Design review of the part built by this model. Coordinates are the model's own, in mm. A direction names the side the tool comes from. Coordinates: 2 decimals unless noted, no trailing zeros. Write each loop counter-clockwise with the first axis right and the second up, starting at its lowest first coordinate (ties: lowest second). Pieces come first, ordered by that corner, then holes. Notation, with made-up numbers: (10.5, 66) -> (30.5, 66) arc R14 ccw to (30.5, 80) -> close; hole circle Ø6 at (31, 52). An arc over 180 degrees is marked (long way). Return JSON: item names as keys, results as strings. Group by question number.
from build123d import *

# Parameters (mm, degrees)
SKETCH2_R                                     = 1.75
CUT_EXTRUDE1_DEPTH                            = 46.369317826
CIRPATTERN1_COUNT                             = 6
SKETCH5_OUTSIDE_W                             = 75.336
SKETCH5_OUTSIDE_H                             = 75.336
SKETCH5_OUTSIDE_R                             = 1.75
CUT_EXTRUDE2_DEPTH                            = 10
CIRPATTERN2_COUNT                             = 6
SKETCH6_R                                     = 12
CUT_EXTRUDE3_DEPTH                            = 4.5
CBORE_FOR_M3_HEX_HEAD_MACHINE_SCREW1_AT_COUNT = 2
CBORE_FOR_M3_HEX_HEAD_MACHINE_SCREW1_AT_PITCH = 23.25
CBORE_FOR_M3_HEX_HEAD_MACHINE_SCREW1_2_COUNT  = 2
CBORE_FOR_M3_HEX_HEAD_MACHINE_SCREW1_2_PITCH  = 40.270181276
CBORE_FOR_M3_HEX_HEAD_MACHINE_SCREW1_3_COUNT  = 2
CBORE_FOR_M3_HEX_HEAD_MACHINE_SCREW1_3_PITCH  = 46.5
CBORE_FOR_M3_HEX_HEAD_MACHINE_SCREW1_4_COUNT  = 2
CBORE_FOR_M3_HEX_HEAD_MACHINE_SCREW1_4_PITCH  = 40.270181276
CBORE_FOR_M3_HEX_HEAD_MACHINE_SCREW1_5_COUNT  = 2
CBORE_FOR_M3_HEX_HEAD_MACHINE_SCREW1_5_PITCH  = 23.25
SKETCH9_R                                     = 4.2
CUT_EXTRUDE4_DEPTH                            = 46.369317826
CIRPATTERN3_START                             = -26.5
CIRPATTERN3_DEPTH                             = 21.5


# Read off the part's stored shape, not the designer's step: CirPattern3
with BuildPart() as part:
    # Sketch1 → Revolve1 (revolve)
    with BuildSketch(Plane(origin=(0, 0, 0), x_dir=(0, 0, -1), z_dir=(1, 0, 0)), mode=Mode.PRIVATE) as revolve1_sk:
        Polygon((0, 0), (0, 28.25), (5, 28.25), (5, 24.5), (8.5, 24.5), (8.5, 22.5), (26.5, 22.5), (26.5, 0), align=None)
    revolve(revolve1_sk.sketch.rotate(Axis((0, 0, 0), (0, 0, -1)), 90), axis=Axis((0, 0, 0), (0, 0, -1)))

    # Sketch2 → Cut-Extrude1 (cut, symmetric)
    with BuildSketch(Plane(origin=(0, 0, -5), x_dir=(-1, 0, 0), z_dir=(0, 0, -1))):
        with Locations((0, 23.25)):
            Circle(SKETCH2_R)
    cut_extrude1 = extrude(amount=CUT_EXTRUDE1_DEPTH, both=True, mode=Mode.SUBTRACT)

    # CirPattern1: Cut-Extrude1 ×6 about axis
    cirpattern1_axis = Axis((0, 0, 0), (0, 0, 1))
    for i in range(1, CIRPATTERN1_COUNT):
        add(cut_extrude1.rotate(cirpattern1_axis, i * 360 / CIRPATTERN1_COUNT), mode=Mode.SUBTRACT)

    # Sketch5 outside → Cut-Extrude2 (cut)
    # profile 1 of 2: a face of its own
    with BuildSketch(Plane(origin=(0, 0, -26.5), x_dir=(-1, 0, 0), z_dir=(0, 0, -1))):
        Rectangle(SKETCH5_OUTSIDE_W, SKETCH5_OUTSIDE_H)
        with BuildLine():
            ThreePointArc((-1.554498096, 22.446236559), (-11.25, 19.485571585), (-18.661762031, 12.569353121))
            ThreePointArc((-18.661762031, 12.569353121), (-18.619546181, 10.75), (-20.216260128, 9.876883438))
            ThreePointArc((-20.216260128, 9.876883438), (-22.5, 0), (-20.216260128, -9.876883438))
            ThreePointArc((-20.216260128, -9.876883438), (-18.619546181, -10.75), (-18.661762031, -12.569353121))
            ThreePointArc((-18.661762031, -12.569353121), (-11.25, -19.485571585), (-1.554498096, -22.446236559))
            ThreePointArc((-1.554498096, -22.446236559), (0, -21.5), (1.554498096, -22.446236559))
            ThreePointArc((1.554498096, -22.446236559), (11.25, -19.485571585), (18.661762031, -12.569353121))
            ThreePointArc((18.661762031, -12.569353121), (18.619546181, -10.75), (20.216260128, -9.876883438))
            ThreePointArc((20.216260128, -9.876883438), (22.5, 0), (20.216260128, 9.876883438))
            ThreePointArc((20.216260128, 9.876883438), (18.619546181, 10.75), (18.661762031, 12.569353121))
            ThreePointArc((18.661762031, 12.569353121), (11.25, 19.485571585), (1.554498096, 22.446236559))
            ThreePointArc((1.554498096, 22.446236559), (0, 21.5), (-1.554498096, 22.446236559))
        make_face(mode=Mode.SUBTRACT)
    # profile 2 of 2: a face of its own
    with BuildSketch(Plane(origin=(0, 0, -26.5), x_dir=(-1, 0, 0), z_dir=(0, 0, -1))):
        with Locations((8.25, 14.289419162)):
            Circle(SKETCH5_OUTSIDE_R)
    cut_extrude2 = extrude(amount=-CUT_EXTRUDE2_DEPTH, mode=Mode.SUBTRACT)

    # CirPattern2: Cut-Extrude2 ×6 about axis
    cirpattern2_axis = Axis((0, 0, 0), (0, 0, 1))
    for i in range(1, CIRPATTERN2_COUNT):
        add(cut_extrude2.rotate(cirpattern2_axis, i * 360 / CIRPATTERN2_COUNT), mode=Mode.SUBTRACT)

    # Sketch6 → Cut-Extrude3 (cut)
    with BuildSketch(Plane.XY):
        Circle(SKETCH6_R)
    extrude(amount=-CUT_EXTRUDE3_DEPTH, mode=Mode.SUBTRACT)

    # Sketch8 → CBORE for M3 Hex Head Machine Screw1 (revolve, cut)
    with BuildSketch(Plane(origin=(20.135090638, 11.625, -5), x_dir=(0, 1, 0), z_dir=(1, 0, 0))):
        Polygon((0, 0), (0, 5), (1.7, 5), (1.7, 2.3), (4.2, 2.3), (4.2, 0), align=None)
    cbore_for_m3_hex_head_machine_screw1 = revolve(axis=Axis((20.135090638, 11.625, -11.35), (0, 0, 1)), mode=Mode.SUBTRACT)

    # CBORE for M3 Hex Head Machine Screw1 at: CBORE for M3 Hex Head Machine Screw1 ×2
    with Locations(*[Vector(-0.8660254037844417, 0.49999999999999484, 0) * (i * CBORE_FOR_M3_HEX_HEAD_MACHINE_SCREW1_AT_PITCH) for i in range(1, CBORE_FOR_M3_HEX_HEAD_MACHINE_SCREW1_AT_COUNT)]):
        add(cbore_for_m3_hex_head_machine_screw1, mode=Mode.SUBTRACT)

    # CBORE for M3 Hex Head Machine Screw1 2: CBORE for M3 Hex Head Machine Screw1 ×2
    with Locations(*[(-i * CBORE_FOR_M3_HEX_HEAD_MACHINE_SCREW1_2_PITCH, 0, 0) for i in range(1, CBORE_FOR_M3_HEX_HEAD_MACHINE_SCREW1_2_COUNT)]):
        add(cbore_for_m3_hex_head_machine_screw1, mode=Mode.SUBTRACT)

    # CBORE for M3 Hex Head Machine Screw1 3: CBORE for M3 Hex Head Machine Screw1 ×2
    with Locations(*[Vector(-0.8660254037844346, -0.5000000000000071, 0) * (i * CBORE_FOR_M3_HEX_HEAD_MACHINE_SCREW1_3_PITCH) for i in range(1, CBORE_FOR_M3_HEX_HEAD_MACHINE_SCREW1_3_COUNT)]):
        add(cbore_for_m3_hex_head_machine_screw1, mode=Mode.SUBTRACT)

    # CBORE for M3 Hex Head Machine Screw1 4: CBORE for M3 Hex Head Machine Screw1 ×2
    with Locations(*[Vector(-0.49999999999999495, -0.8660254037844416, 0) * (i * CBORE_FOR_M3_HEX_HEAD_MACHINE_SCREW1_4_PITCH) for i in range(1, CBORE_FOR_M3_HEX_HEAD_MACHINE_SCREW1_4_COUNT)]):
        add(cbore_for_m3_hex_head_machine_screw1, mode=Mode.SUBTRACT)

    # CBORE for M3 Hex Head Machine Screw1 5: CBORE for M3 Hex Head Machine Screw1 ×2
    with Locations(*[(0, -i * CBORE_FOR_M3_HEX_HEAD_MACHINE_SCREW1_5_PITCH, 0) for i in range(1, CBORE_FOR_M3_HEX_HEAD_MACHINE_SCREW1_5_COUNT)]):
        add(cbore_for_m3_hex_head_machine_screw1, mode=Mode.SUBTRACT)

    # Sketch9 → Cut-Extrude4 (cut, through all)
    with BuildSketch(Plane(origin=(0, 0, -5), x_dir=(-1, 0, 0), z_dir=(0, 0, -1))):
        with Locations((-20.135090638, 11.625)):
            Circle(SKETCH9_R)
    extrude(amount=CUT_EXTRUDE4_DEPTH, mode=Mode.SUBTRACT)

    # CirPattern3 outline → CirPattern3 (cut)
    with BuildSketch(Plane.XY.offset(CIRPATTERN3_START)):
        with BuildLine():
            ThreePointArc((-1.256823209, 24.467741935), (-2.811398825, 24.338160091), (-4.35457664, 24.109907969))
            ThreePointArc((-4.35457664, 24.109907969), (-0.179741778, 19.176685596), (3.901890218, 24.187295275))
            ThreePointArc((3.901890218, 24.187295275), (2.58316543, 24.363440979), (1.256823209, 24.467741935))
            ThreePointArc((1.256823209, 24.467741935), (0, 21.5), (-1.256823209, 24.467741935))
        make_face()
        with BuildLine():
            ThreePointArc((-18.968503996, 15.506316654), (-19.795032609, 14.436297449), (-20.561274485, 13.322311795))
            ThreePointArc((-20.561274485, 13.322311795), (-18.619546181, 10.75), (-21.818097694, 11.145430141))
            ThreePointArc((-21.818097694, 11.145430141), (-22.490778714, 9.716731593), (-23.070024017, 8.247665844))
            ThreePointArc((-23.070024017, 8.247665844), (-16.916681459, 9.558816026), (-18.968503996, 15.506316654))
        make_face()
        with BuildLine():
            ThreePointArc((-21.818097694, -11.145430141), (-18.619546181, -10.75), (-20.561274485, -13.322311795))
            ThreePointArc((-20.561274485, -13.322311795), (-19.723759912, -14.533523143), (-18.81499127, -15.692230674))
            ThreePointArc((-18.81499127, -15.692230674), (-16.935996673, -9.778002238), (-22.997366041, -8.448145074))
            ThreePointArc((-22.997366041, -8.448145074), (-22.448280204, -9.814515571), (-21.818097694, -11.145430141))
        make_face()
        with BuildLine():
            ThreePointArc((-1.256823209, -24.467741935), (0, -21.5), (1.256823209, -24.467741935))
            ThreePointArc((1.256823209, -24.467741935), (2.604684023, -24.361149832), (3.944612144, -24.180364659))
            ThreePointArc((3.944612144, -24.180364659), (-0.18016322, -19.429683905), (-4.392323866, -24.103059786))
            ThreePointArc((-4.392323866, -24.103059786), (-2.830452956, -24.335951513), (-1.256823209, -24.467741935))
        make_face()
        with BuildLine():
            ThreePointArc((20.561274485, -13.322311795), (18.619546181, -10.75), (21.818097694, -11.145430141))
            ThreePointArc((21.818097694, -11.145430141), (22.390941527, -9.944633606), (22.897757266, -8.714511586))
            ThreePointArc((22.897757266, -8.714511586), (16.517625997, -9.744003743), (18.702504464, -15.826127977))
            ThreePointArc((18.702504464, -15.826127977), (19.671765509, -14.603822849), (20.561274485, -13.322311795))
        make_face()
    extrude(amount=CIRPATTERN3_DEPTH, mode=Mode.SUBTRACT)


solid = part.part
Q1. For faces 4 (the flat face through (-23, 0, -8.5)), 5 (the flat face through (11, 20, -8.5)), 6 (the cylindrical face through (16.57, -9.66, -15.9)), 7 (the cylindrical face through (-11.267, -19.476, -17.626)), list the 3-axis set-ups (+Z, -Z, +X, -X, +Y, -Y) from which the entire face can be reached by the end or side of a thin tool; tool diameter is ignored.
Q2. We need section A-A on y = -23.25. Write out the cut boundary in (x, z).
Q3. We need section C-C on z = -23. State how many separate pieces and enclosed holes the cut face has, plus the area to 3 significant figures.
Q4. We need section D-D on x = -8.25. Write out the cut boundary in (y, z), plus the area to 3 significant figures.
Q5. For P1, Ø4, axis at y = -21.5, z = -22.5, coming from the -X side (3 decimals); P2, Ø12, axis at x = -0.5, y = -1, coming from the +Z side; P3, Ø4, axis at x = -1, y = -22, coming from the -Z side; P4, Ø2, axis at x = 20.14, y = 11.63, coming from the -Z side, all flat-tipped, find the tip position at first contact; note any pin that passes through.
Q6. We need section B-B on y = 0. Write out the cut boundary in (x, z), plus the area to 3 significant figures.
Q7. The part is to be moulded in two halves that separate along Z. For faces 1 (the flat face through (-16.2, 11.5, -5)), 2 (the cylindrical face through (6.9, 15.4, -21.6)), 3 (the flat face through (-12.2, -0.4, 0)), say which applies: +Z half, -Z half, draft (parallel to the pull), parting line (faces both ways), or undercut.
Q8. Wall thickness on L1, parallel to X at y = -23.25, z = -4; L2, parallel to Y at x = -8.25, z = -21.75; L3, parallel to X at y = 14, z = -18.5: over which ranges is each line inside the solid? List them lowest first.
Findings below:
{
 "1": {"face 4": "-Z, -X", "face 5": "-Z, +X, +Y", "face 6": "-Z", "face 7": "-Z, -X, -Y"},
 "2": {"outline": "(-16.05, -5) -> (-7.73, -5) -> (-7.73, -8.5) -> (-4.4, -8.5) -> (-4.4, -5) -> (-4.2, -5) -> (-4.2, -2.7) -> (-1.75, -2.7) -> (-1.75, 0) -> (-16.05, 0) -> close; (1.75, -2.7) -> (4.2, -2.7) -> (4.2, -5) -> (3.96, -5) -> (3.96, -8.5) -> (7.73, -8.5) -> (7.73, -5) -> (16.05, -5) -> (16.05, 0) -> (1.75, 0) -> close"},
 "3": {"separate pieces": "1", "enclosed holes": "6", "area": "1,420 mm^2"},
 "4": {"outline": "(-27.02, -5) -> (-23.07, -5) -> (-23.07, -8.5) -> (-20.93, -8.5) -> (-20.93, -26.5) -> (-16.04, -26.5) -> (-16.04, -16.5) -> (-12.54, -16.5) -> (-12.54, -26.5) -> (12.54, -26.5) -> (12.54, -16.5) -> (16.04, -16.5) -> (16.04, -26.5) -> (20.93, -26.5) -> (20.93, -8.5) -> (23.07, -8.5) -> (23.07, -5) -> (27.02, -5) -> (27.02, 0) -> (8.71, 0) -> (8.71, -4.5) -> (-8.71, -4.5) -> (-8.71, 0) -> (-27.02, 0) -> close", "area": "1,040 mm^2"},
 "5": {"P1": "stops at x = -11.225", "P2": "stops at z = -4.5", "P3": "stops at z = -2.7", "P4": "passes through"},
 "6": {"outline": "(-28.25, -5) -> (-24.5, -5) -> (-24.5, -8.5) -> (-22.5, -8.5) -> (-22.5, -26.5) -> (-18.25, -26.5) -> (-18.25, -16.5) -> (-14.75, -16.5) -> (-14.75, -26.5) -> (14.75, -26.5) -> (14.75, -16.5) -> (18.25, -16.5) -> (18.25, -26.5) -> (22.5, -26.5) -> (22.5, -8.5) -> (24.5, -8.5) -> (24.5, -5) -> (28.25, -5) -> (28.25, 0) -> (12, 0) -> (12, -4.5) -> (-12, -4.5) -> (-12, 0) -> (-28.25, 0) -> close", "area": "1,090 mm^2"},
 "7": {"face 1": "undercut", "face 2": "draft", "face 3": "+Z half"},
 "8": {"L1": "x = -16.05 to -4.2, 4.2 to 16.05", "L2": "y = -20.93 to -16.04, -12.54 to 12.54, 16.04 to 20.93", "L3": "x = -17.11 to -9.98, -6.52 to 6.52, 9.98 to 16.67"}
}
